Source: CAD feature listing. Evaluate the final solid. Frame: model axes, mm. Face numbers are marked on the shaded views. A direction names the side the tool comes from. Coordinates: 2 decimals unless noted, no trailing zeros. Write each loop counter-clockwise with the first axis right and the second up, starting at its lowest first coordinate (ties: lowest second). Pieces come first, ordered by that corner, then holes. Notation, with made-up numbers: M 67.5,-22.75 L 87.5,-22.75 A28 cw 87.5,13.25 Z; hole C 16.5,-17.5 d7. An arc over 180 degrees is marked long. Answer as CSV lines item,"result". Start each with the question number.
1. Section D-D on x = -13. Return the cut outline in (y, z).
2. Line query: probe 1 along X at (y, z) = (2, -15); probe 2 along X at (y, z) = (2.5, 10); probe 3 along X at (y, z) = (3.5, 0). Output: solid intervals per line, ascending. Write a range as [from, to].
3. Contact query for flat-ended pins moving along their axis: pin 1 Ø3.5 at (x, z) = (20, -15) entering from +Y; pin 2 Ø1.5 at (x, z) = (9.5, 7.5) entering from +Y; pin 3 Ø10 at (x, z) = (-19, 14) entering from -Y; pin 4 Ø6.5 at (x, y) = (20, -12) entering from -Z. Output: stop coordinate, or through.
4. Section C-C on x = 0. Return the cut outline in (y, z).
5. Section A-A on z = 0. Return the cut outline in (x, y), plus the area to 3 significant figures.
6. Section B-B on x = 20. Return the cut outline in (y, z), plus the area to 3 significant figures.
7. Reachability of the marked faces 1, 2 and 3 from +Z, -Z, +X, -X, +Y, -Y: full face, straight path, thin tool, end or side. Return the list, or none.
8. Mould query, pull axis X, two halves, no side actions, for the marked faces 4, 5 and 6. Classes: pulls with the +X half, pulls with the -X half, needs draft (parallel to the pull), parting line crosses it, or undercut.
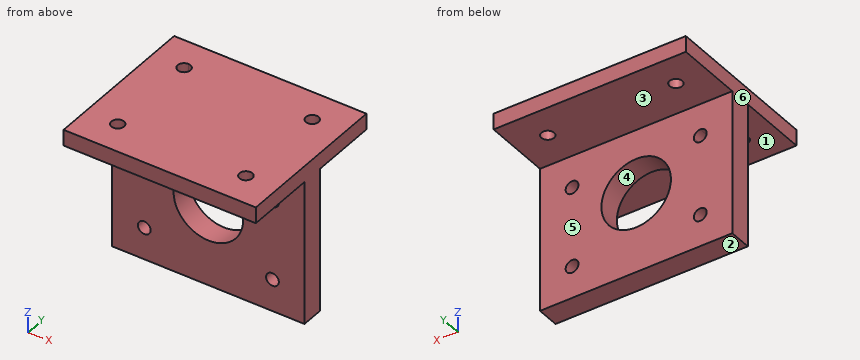
```python
from build123d import *

# Parameters (mm, degrees)
SKETCH_2_W          = 60
SKETCH_2_H          = 50
SKETCH_2_R          = 10.85
EXTRUDE_1_DEPTH     = 7
SKETCH_4_W          = 60
SKETCH_4_H          = 5
EXTRUDE_2_DEPTH     = 25
SKETCH_6_R          = 2
CUT_EXTRUDE_1_DEPTH = 50
SKETCH_8_R          = 2
CUT_EXTRUDE_4_DEPTH = 50


with BuildPart() as part:
    # 草图2 → 凸台-拉伸1 (new body)
    with BuildSketch(Plane(origin=(0, 0, 0), x_dir=(1, 0, 0), z_dir=(0, 1, 0))):
        Rectangle(SKETCH_2_W, SKETCH_2_H)
        with Locations(Location((0, 0, 0), (0, 0, 270))):
            Circle(SKETCH_2_R, mode=Mode.SUBTRACT)
    extrude(amount=EXTRUDE_1_DEPTH)

    # 草图4 → 凸台-拉伸2 (add, symmetric)
    with BuildSketch(Plane(origin=(0, 3, 0), x_dir=(1, 0, 0), z_dir=(0, 1, 0))):
        with Locations((0, -22.5)):
            Rectangle(SKETCH_4_W, SKETCH_4_H)
    extrude(amount=EXTRUDE_2_DEPTH, both=True)

    # 草图6 → 切除-拉伸1 (cut)
    with BuildSketch(Plane.XY.offset(25)):
        with BuildLine():
            ThreePointArc((-18, 18), (-18.585786438, 19.414213562), (-20, 20))
            Line((-20, 20), (-20, 18))
            Line((-20, 18), (-22, 18))
            ThreePointArc((-22, 18), (-20, 16), (-18, 18))
        make_face()
        with BuildLine():
            Line((-20, 18), (-20, 20))
            ThreePointArc((-20, 20), (-21.414213562, 19.414213562), (-22, 18))
            Line((-22, 18), (-20, 18))
        make_face()
        with Locations((20, 18)):
            Circle(SKETCH_6_R)
        with Locations((-20, -12)):
            Circle(SKETCH_6_R)
        with Locations((20, -12)):
            Circle(SKETCH_6_R)
    extrude(amount=-CUT_EXTRUDE_1_DEPTH, mode=Mode.SUBTRACT)

    # 草图8 → 切除-拉伸4 (cut)
    with BuildSketch(Plane.XZ):
        with BuildLine():
            ThreePointArc((-18, 10), (-18.585786438, 11.414213562), (-20, 12))
            Line((-20, 12), (-20, 10))
            Line((-20, 10), (-22, 10))
            ThreePointArc((-22, 10), (-20, 8), (-18, 10))
        make_face()
        with BuildLine():
            Line((-20, 10), (-20, 12))
            ThreePointArc((-20, 12), (-21.414213562, 11.414213562), (-22, 10))
            Line((-22, 10), (-20, 10))
        make_face()
        with Locations(Location((20, 10, 0), (0, 0, 270))):
            Circle(SKETCH_8_R)
        with Locations(Location((20, -15, 0), (0, 0, 270))):
            Circle(SKETCH_8_R)
        with Locations(Location((-20, -15, 0), (0, 0, 270))):
            Circle(SKETCH_8_R)
    extrude(amount=-CUT_EXTRUDE_4_DEPTH, mode=Mode.SUBTRACT)


solid = part.part
```
Values:
1,outline,"M -22,20 L 0,20 L 0,-25 L 7,-25 L 7,20 L 28,20 L 28,25 L -22,25 Z"
2,probe 1,"[-30, -22], [-18, 18], [22, 30]"
2,probe 2,"[-30, -22], [-18, -4.21], [4.21, 18], [22, 30]"
2,probe 3,"[-30, -10.85], [10.85, 30]"
3,pin 1,"through"
3,pin 2,"y = 7"
3,pin 3,"y = 0"
3,pin 4,"z = 20"
4,outline,"M -22,20 L 0,20 L 0,10.85 L 7,10.85 L 7,20 L 28,20 L 28,25 L -22,25 Z; M 0,-25 L 7,-25 L 7,-10.85 L 0,-10.85 Z"
5,outline,"M -30,0 L -10.85,0 L -10.85,7 L -30,7 Z; M 10.85,0 L 30,0 L 30,7 L 10.85,7 Z"
5,area,"268 mm²"
6,outline,"M -22,20 L -14,20 L -14,25 L -22,25 Z; M -10,20 L 0,20 L 0,12 L 7,12 L 7,20 L 16,20 L 16,25 L -10,25 Z; M 0,-25 L 7,-25 L 7,-17 L 0,-17 Z; M 0,-13 L 7,-13 L 7,8 L 0,8 Z; M 20,20 L 28,20 L 28,25 L 20,25 Z"
6,area,"469 mm²"
7,face 1,"-Z, +X, -X, -Y"
7,face 2,"-Z, +X, -X, +Y, -Y"
7,face 3,"-Z, +X, -X, +Y"
8,face 4,"undercut"
8,face 5,"needs draft"
8,face 6,"pulls with the -X half"
